CAD build for the part. Positions are in the model's coordinates, mm. A direction names the side the tool comes from. Give positions to 0.01 mm unless a question says otherwise; leave off trailing zeros. Order: outer loops, then holes, each group sorted by start corner. A loop starts at its lowest first (then second) coordinate and runs counter-clockwise, first axis right, second up. Notation, with made-up numbers: (68.5, 16) -> (110.5, 16) arc R16 ccw to (110.5, 46) -> close; hole circle Ø10 at (34.25, 81). An arc over 180 degrees is marked (long way). Use one line per item in the form item = value. Start each with the question number.
1) Cut at B-B, the plane z = 29.5. Give the cut face in (x, y), and give its area (3 significant figures).
2) Cut at C-C, the plane y = 1.1. State how many separate pieces and enclosed holes the cut face has, and give its area (3 significant figures).
3) Mould opens along X. For faces 1 (the face through (31.48, 0.99, 46.55)), 2 (the face through (-37, 1, 33.6)), 3 (the face through (37.81, 0.99, -35.38)) say: pulls with the +X half, pulls with the -X half, needs draft (parallel to the pull), parting line crosses it, or undercut.
4) Drop a flat-ended pin along its axis: P1, Ø1, axis at x = -24.5, y = 1.5, coming from the +Z side. Give the stop position or say it passes through.
5) Probe line 1 (X direction, y = 0.2, z = 3); line 2 (Z direction, x = -7, y = 0.65); line 3 (X direction, y = 1.3, z = 7.5). List the from-to ranges inside material, lowest first.
6) Tool access for faces 4 (the face through (9.5, 0, 0.4)), 5 (the face through (-24.166, 0.986, 31.534)): list every direction of +Z, -Z, +X, -X, +Y, -Y with a clear straight run to the whole face (end or side of a thin tool).
7) Cut at A-A, the plane z = 0. Give the cut face in (x, y).
from build123d import *

# Parameters (mm, degrees)
SKETCH_1_R          = 1.5
SKETCH_1_R_2        = 4
EXTRUDE_1_DEPTH     = 2
SKETCH_2_R          = 1.5
CUT_EXTRUDE_1_DEPTH = 116.094668721


with BuildPart() as part:
    # Эскиз1 → Бобышка-Вытянуть1 (new body)
    with BuildSketch(Plane(origin=(0, 0, 0), x_dir=(1, 0, 0), z_dir=(0, 1, 0))):
        with BuildLine():
            Line((54.236033393, -5.45028137), (20.920510558, 77.368874006))
            add(Edge.make_bspline(
                [(20.920510558, 77.368874006), (13.519104954, 99.996768719), (0, 100)],
                knots=[2.149983836, 2.149983836, 2.149983836, 3.14143331, 3.14143331, 3.14143331], degree=2, weights=[1, 0.879624206, 1]))
            Line((0, 100), (0, 93))
            add(Edge.make_bspline(
                [(18.005142203, 50.270253613), (17.382191681, 91.773168681), (0, 93)],
                knots=[1.570796327, 1.570796327, 1.570796327, 3.105746544, 3.105746544, 3.105746544], degree=2, weights=[1, 0.719666045, 1]))
            add(Edge.make_bspline(
                [(-13.452394346, 7.504043857), (16.003264405, 13.845732338), (18.005142203, 50.270253613)],
                knots=[0, 0, 0, 1, 1, 1], degree=2))
            ThreePointArc((-13.452394346, 7.504043857), (-36.870731242, -34.340992448), (0, -65))
            ThreePointArc((0, -65), (24.874423104, -60.052169613), (45.961940777, -45.961940777))
            ThreePointArc((45.961940777, -45.961940777), (56.186949809, -26.949515273), (54.236033393, -5.45028137))
        make_face()
        with Locations(Location((9.550649772, -54.164426416, 0), (0, 0, 270))):
            Circle(SKETCH_1_R, mode=Mode.SUBTRACT)
        with Locations(Location((31.546703999, -45.053362436, 0), (0, 0, 90))):
            Circle(SKETCH_1_R, mode=Mode.SUBTRACT)
        with Locations(Location((0, 0, 0), (0, 0, 270))):
            Circle(SKETCH_1_R_2, mode=Mode.SUBTRACT)
        with Locations(Location((0, -7.5, 0), (0, 0, 270))):
            Circle(SKETCH_1_R, mode=Mode.SUBTRACT)
        with Locations(Location((0, 7.5, 0), (0, 0, 270))):
            Circle(SKETCH_1_R, mode=Mode.SUBTRACT)
        with BuildLine():
            ThreePointArc((0, -52), (19.899538483, -48.041735691), (36.769552622, -36.769552622))
            ThreePointArc((36.769552622, -36.769552622), (39.657964622, -5.59972573), (9.54966327, 2.967141962))
            ThreePointArc((9.54966327, 2.967141962), (7.071067812, -7.071067812), (-2.967141962, -9.54966327))
            ThreePointArc((-2.967141962, -9.54966327), (-6.395779647, -7.687262368), (-8.850717859, -4.654545455))
            ThreePointArc((-8.850717859, -4.654545455), (-24.082811675, -32.002019749), (0, -52))
        make_face(mode=Mode.SUBTRACT)
    extrude(amount=EXTRUDE_1_DEPTH)

    # Эскиз2 → Вырез-Вытянуть1 (cut, through all)
    with BuildSketch(Plane.XZ):
        with Locations(Location((3.997292475, -95.689262056, 0), (0, 0, 270))):
            Circle(SKETCH_2_R)
        with Locations(Location((10.780229305, -90.232363482, 0), (0, 0, 270))):
            Circle(SKETCH_2_R)
    extrude(amount=-CUT_EXTRUDE_1_DEPTH, mode=Mode.SUBTRACT)


solid = part.part
Result:
q1.outline = (-37.45, 0) -> (-24.42, 0) -> (-24.42, 2) -> (-37.45, 2) -> close; (41.79, 0) -> (55.57, 0) -> (55.57, 2) -> (41.79, 2) -> close
q1.area = 53.6 mm²
q2.separate_pieces = 1
q2.enclosed_holes = 8
q2.area = 4,480 mm²
q3.face_1 = undercut
q3.face_2 = pulls with the -X half
q3.face_3 = pulls with the +X half
q4.P1 = 56.31
q5.line_1 = -28.39 to -2.65, 2.65 to 9.54, 37.61 to 53.25
q5.line_2 = -9.38 to 7.14, 50.98 to 64.34
q5.line_3 = -31.72 to -14.15, -6.61 to -1.5, 1.5 to 6.61, 40.84 to 54.99
q6.face_4 = +Z, -Z, +X, -X, -Y
q6.face_5 = +Y, -Y
q7.outline = (-25.5, 0) -> (-4, 0) -> (-4, 2) -> (-25.5, 2) -> close; (4, 0) -> (10, 0) -> (10, 2) -> (4, 2) -> close; (34.35, 0) -> (52.04, 0) -> (52.04, 2) -> (34.35, 2) -> close
